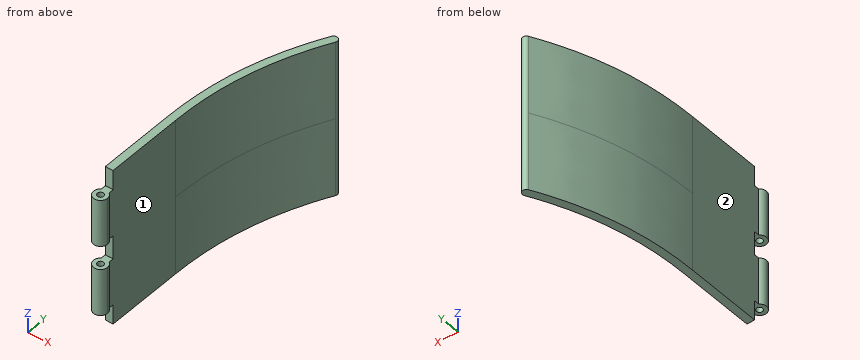
```python
from build123d import *

# Parameters (mm, degrees)
BOSS_EXTRUDE1_DEPTH = 50
BOSS_EXTRUDE2_START = -12.5
SKETCH2_R           = 2
BOSS_EXTRUDE2_DEPTH = 30


with BuildPart() as part:
    # Sketch1 → Boss-Extrude1 (new body, symmetric)
    with BuildSketch(Plane.XY):
        with BuildLine():
            Line((0, 0), (0, 50))
            add(Edge.make_bspline(
                [(0, 50), (-0.236079675, 103.300249741), (25, 150)],
                knots=[0, 0, 0, 1, 1, 1], degree=2))
            ThreePointArc((25, 150), (28.387941146, 151.010868336), (29.398809482, 147.62292719))
            add(Edge.make_bspline(
                [(5, 50.011073049), (4.990421387, 52.173658537), (5.035623154, 56.511554686), (5.385764781, 65.083196163), (6.308823956, 75.675961605), (8.192566934, 88.173154483), (10.852002898, 100.466008633), (14.287860292, 112.557101091), (18.500659336, 124.449247631), (22.66257211, 134.200371846), (26.379067858, 141.898054896), (28.374986615, 145.728327364), (29.398809482, 147.62292719)],
                knots=[-0.000103873, -0.000103873, -0.000103873, -0.000103873, 0.062402619, 0.124909111, 0.249922095, 0.374935079, 0.499948063, 0.624961048, 0.749974032, 0.874987016, 0.937493508, 1, 1, 1, 1], degree=3))
            Line((5, 50.011073049), (5, 0))
            Line((5, 0), (0, 0))
        make_face()
    extrude(amount=BOSS_EXTRUDE1_DEPTH, both=True)

    # Sketch2 → Boss-Extrude2 (add)
    with BuildSketch(Plane.XY.offset(50).offset(BOSS_EXTRUDE2_START)):
        with BuildLine():
            Line((5, -3.258342613), (0, -3.258342613))
            ThreePointArc((0, -3.258342613), (0.378679656, -10.968626967), (7, -7))
            ThreePointArc((7, -7), (6.468626967, -4.878679656), (5, -3.258342613))
        make_face()
        with Locations((2.5, -7)):
            Circle(SKETCH2_R, mode=Mode.SUBTRACT)
        with BuildLine():
            ThreePointArc((5, -3.258342613), (2.5, -2.5), (0, -3.258342613))
            Line((0, -3.258342613), (5, -3.258342613))
        make_face()
        with BuildLine():
            Line((5, 0), (0, 0))
            Line((0, 0), (0, -3.258342613))
            ThreePointArc((0, -3.258342613), (2.5, -2.5), (5, -3.258342613))
            Line((5, -3.258342613), (5, 0))
        make_face()
    boss_extrude2 = extrude(amount=-BOSS_EXTRUDE2_DEPTH)

    # Mirror1: Boss-Extrude2 across plane
    add(boss_extrude2.mirror(Plane.XY))


solid = part.part
```
Here's how the part is built. I have some questions about the finished solid (model axes, mm). Face numbers are marked on the shaded views. Give positions to 0.01 mm unless a question says otherwise; leave off trailing zeros. Order: outer loops, then holes, each group sorted by start corner. A loop starts at its lowest first (then second) coordinate and runs counter-clockwise, first axis right, second up. Notation, with made-up numbers: M -22,0 L 0,0 A22 cw 0,21 Z; hole C 47.25,30.25 d10. An arc over 180 degrees is marked long. Use a Markdown table: item, result. Add a question column.
1. I need wall thicknesses on probe 1 along X at (y, z) = (32.5, -1); probe 2 along Y at (x, z) = (24.5, -18.5); probe 3 along X at (y, z) = (68, -42). Which ranges of each line are inside material? Lowest first, please. Write a range as from..to.
2. Suppose I cut it at B-B (y = 37). List the corners of the cut face in (x, z) for me.
3. If we mould it in two halves opening along Y, with no side actions, what happens to the marked faces 1 and 2? For each: +Y half, -Y half, draft (parallel to the pull), parting line (faces both ways), or undercut.
4. Suppose I cut it at A-A (x = 2.5). Give the number of separate pieces and of enclosed holes in the cut face, and give its area (3 significant figures).
5. For pin 1 Ø4 at (x, z) = (3.5, 46) entering from -Y; pin 2 Ø1.5 at (y, z) = (33, -37.5) entering from -X; pin 3 Ø1 at (y, z) = (131, 28.5) entering from -X, each with a flat end and sliding along its axis, tell me the tip position at first contact or that it passes through.
Results list:
| question | item | result |
|---|---|---|
| 1 | probe 1 | x = 0..5 |
| 1 | probe 2 | y = 137.98..149.07 |
| 1 | probe 3 | x = 0.66..5.68 |
| 2 | outline | M 0,-50 L 5,-50 L 5,50 L 0,50 Z |
| 3 | face 1 | undercut |
| 3 | face 2 | draft |
| 4 | separate pieces | 3 |
| 4 | enclosed holes | 0 |
| 4 | area | 8,820 mm² |
| 5 | pin 1 | stops at y = 0 |
| 5 | pin 2 | stops at x = 0 |
| 5 | pin 3 | stops at x = 15.69 |
